Input: dimensioned drawing with shaded views. Units: mm. Origin: part minimum x, y, z. A direction names the side the tool comes from. Coordinates: 2 decimals unless noted, no trailing zeros. Loops run counter-clockwise (first coordinate to the right, second up) from the corner with the lowest first, then second, coordinate; pieces in that order, holes last.
Item 1: Section query A-A, the plane y = 11.5. Return the cut outline in (x, z) (1 decimal).
Item 2: Section query C-C, the plane x = 3.25. Return the cut outline in (y, z) (1 decimal).
Item 3: Line query: probe 1 along X at (y, z) = (4.5, 2.75) (1 decimal); probe 2 along Y at (x, z) = (12.5, 5.5) (1 decimal). Output: solid intervals per line, ascending.
Item 4: Pull-direction query (Y, two-part tool) for the marked faces 4, 5 and 6; classes: +Y half, -Y half, draft (parallel to the pull), parting line (faces both ways), or undercut.
Item 5: Section query D-D, the plane x = 10.5. Return the cut outline in (y, z).
Item 6: Reachability of the marked faces 1, 2 and 3 from +Z, -Z, +X, -X, +Y, -Y: full face, straight path, thin tool, end or side. Return the list, or none.
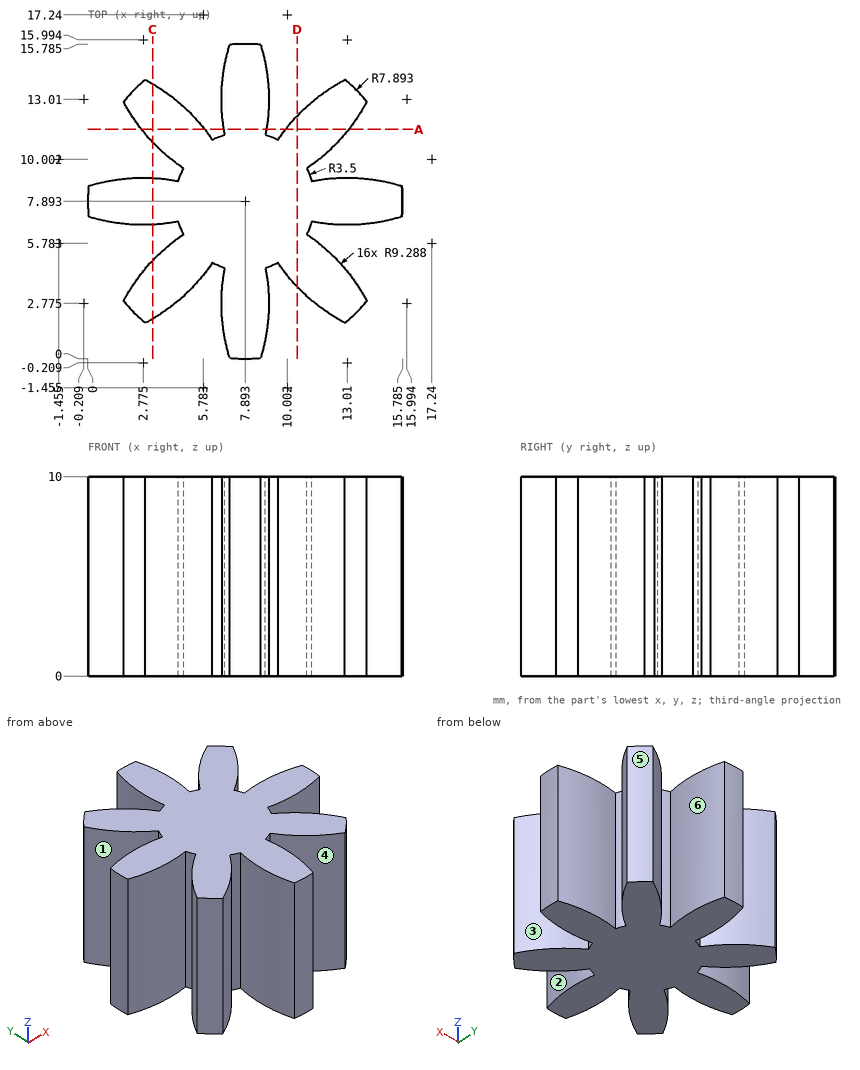
Verdict:
1. outline: (2.7, 0) - (5.9, 0) - (5.9, 10) - (2.7, 10) - close; (6.8, 0) - (9, 0) - (9, 10) - (6.8, 10) - close; (9.9, 0) - (13.1, 0) - (13.1, 10) - (9.9, 10) - close
2. outline: (2, 0) - (4.9, 0) - (4.9, 10) - (2, 10) - close; (6.7, 0) - (9.1, 0) - (9.1, 10) - (6.7, 10) - close; (10.9, 0) - (13.8, 0) - (13.8, 10) - (10.9, 10) - close
3. probe 1: x = 2.9 to 6, 6.9 to 8.9, 9.8 to 12.9
3. probe 2: y = 2 to 5, 6.7 to 9.1, 10.8 to 13.8
4. face 4: -Y half
4. face 5: +Y half
4. face 6: undercut
5. outline: (3.61, 0) - (12.17, 0) - (12.17, 10) - (3.61, 10) - close
6. face 1: +Z, -Z, -X
6. face 2: +Z, -Z
6. face 3: +Z, -Z, +X
